from build123d import *

# Parameters (mm, degrees)
F0_R        = 72.39
F1_DEPTH    = 6.35
F2_DEPTH    = 50.8
F3_T1_DEPTH = 69.85
F5_DEPTH    = 31.75


# Not quite as in the source:
# - a fillet or chamfer that OpenCascade refuses, or shapes differently, is made with other operations: its cross-section is extruded or revolved along the edge and cut away or added


with BuildPart() as f1:
    # F0 (on Top) → F1 (new body)
    with BuildSketch(Plane.XY):
        with BuildLine():
            Line((38.1, -87.9881810245), (50.8, -87.9881810245))
            Line((50.8, -87.9881810245), (57.15, -76.9896583964))
            ThreePointArc((57.15, -76.9896583964), (109.1955678842, -63.0440905122), (95.25, -10.9985226281))
            Line((95.25, -10.9985226281), (101.6, 0))
            Line((101.6, 0), (95.25, 10.9985226281))
            ThreePointArc((95.25, 10.9985226281), (109.1955678842, 63.0440905122), (57.15, 76.9896583964))
            Line((57.15, 76.9896583964), (50.8, 87.9881810245))
            Line((50.8, 87.9881810245), (38.1, 87.9881810245))
            ThreePointArc((38.1, 87.9881810245), (0, 126.0881810245), (-38.1, 87.9881810245))
            Line((-38.1, 87.9881810245), (-50.8, 87.9881810245))
            Line((-50.8, 87.9881810245), (-57.15, 76.9896583964))
            ThreePointArc((-57.15, 76.9896583964), (-109.1955678842, 63.0440905122), (-95.25, 10.9985226281))
            Line((-95.25, 10.9985226281), (-101.6, 0))
            Line((-101.6, 0), (-95.25, -10.9985226281))
            ThreePointArc((-95.25, -10.9985226281), (-109.1955678842, -63.0440905122), (-57.15, -76.9896583964))
            Line((-57.15, -76.9896583964), (-50.8, -87.9881810245))
            Line((-50.8, -87.9881810245), (-38.1, -87.9881810245))
            ThreePointArc((-38.1, -87.9881810245), (0, -126.0881810245), (38.1, -87.9881810245))
        make_face()
        Circle(F0_R, mode=Mode.SUBTRACT)
    extrude(amount=F1_DEPTH)

    # F0 (on Top) → F2 (join)
    with BuildSketch(Plane.XY):
        Circle(F0_R)
    extrude(amount=F2_DEPTH)

    # F3: fillet of radius 38.1 on 6 edges, made by hand

    # F3_s2 → F3_t1 (cut)
    with BuildSketch(Plane.XY.offset(-31.75)):
        with BuildLine():
            ThreePointArc((57.15, 76.9896583964), (48.4360135972, 83.8936364665), (38.1, 87.9881810245))
            Line((38.1, 87.9881810245), (50.8, 87.9881810245))
            Line((50.8, 87.9881810245), (57.15, 76.9896583964))
        make_face()
        with BuildLine():
            ThreePointArc((95.25, -10.9985226281), (96.8720271945, 0), (95.25, 10.9985226281))
            Line((95.25, 10.9985226281), (101.6, 0))
            Line((101.6, 0), (95.25, -10.9985226281))
        make_face()
        with BuildLine():
            ThreePointArc((38.1, -87.9881810245), (48.4360135972, -83.8936364665), (57.15, -76.9896583964))
            Line((57.15, -76.9896583964), (50.8, -87.9881810245))
            Line((50.8, -87.9881810245), (38.1, -87.9881810245))
        make_face()
        with BuildLine():
            ThreePointArc((-38.1, -87.9881810245), (-48.4360135972, -83.8936364665), (-57.15, -76.9896583964))
            Line((-57.15, -76.9896583964), (-50.8, -87.9881810245))
            Line((-50.8, -87.9881810245), (-38.1, -87.9881810245))
        make_face()
        with BuildLine():
            ThreePointArc((-95.25, 10.9985226281), (-96.8720271945, 0), (-95.25, -10.9985226281))
            Line((-95.25, -10.9985226281), (-101.6, 0))
            Line((-101.6, 0), (-95.25, 10.9985226281))
        make_face()
        with BuildLine():
            ThreePointArc((-38.1, 87.9881810245), (-48.4360135972, 83.8936364665), (-57.15, 76.9896583964))
            Line((-57.15, 76.9896583964), (-50.8, 87.9881810245))
            Line((-50.8, 87.9881810245), (-38.1, 87.9881810245))
        make_face()
    extrude(amount=F3_T1_DEPTH, mode=Mode.SUBTRACT)

    # F4 (on face) → F5 (join)
    with BuildSketch(Plane.XY.offset(6.35)):
        with BuildLine():
            ThreePointArc((-95.25, -10.9985226281), (-109.1955678842, -63.0440905122), (-57.15, -76.9896583964))
            ThreePointArc((-57.15, -76.9896583964), (-48.4360135972, -83.8936364665), (-38.1, -87.9881810245))
            ThreePointArc((-38.1, -87.9881810245), (0, -126.0881810245), (38.1, -87.9881810245))
            ThreePointArc((38.1, -87.9881810245), (48.4360135972, -83.8936364665), (57.15, -76.9896583964))
            ThreePointArc((57.15, -76.9896583964), (109.1955678842, -63.0440905122), (95.25, -10.9985226281))
            ThreePointArc((95.25, -10.9985226281), (96.8720271945, 0), (95.25, 10.9985226281))
            ThreePointArc((95.25, 10.9985226281), (109.1955678842, 63.0440905122), (57.15, 76.9896583964))
            ThreePointArc((57.15, 76.9896583964), (48.4360135972, 83.8936364665), (38.1, 87.9881810245))
            ThreePointArc((38.1, 87.9881810245), (0, 126.0881810245), (-38.1, 87.9881810245))
            ThreePointArc((-38.1, 87.9881810245), (-48.4360135972, 83.8936364665), (-57.15, 76.9896583964))
            ThreePointArc((-57.15, 76.9896583964), (-109.1955678842, 63.0440905122), (-95.25, 10.9985226281))
            ThreePointArc((-95.25, 10.9985226281), (-96.8720271945, 0), (-95.25, -10.9985226281))
        make_face()
        with BuildLine():
            ThreePointArc((-92.7564557809, 13.2428401804), (-106.4459372272, 61.4565905122), (-57.8468639049, 73.7080269811))
            ThreePointArc((-57.8468639049, 73.7080269811), (-46.8485135972, 81.1440058095), (-34.909591876, 86.9508671615))
            ThreePointArc((-34.909591876, 86.9508671615), (0, 122.9131810245), (34.909591876, 86.9508671615))
            ThreePointArc((34.909591876, 86.9508671615), (46.8485135972, 81.1440058095), (57.8468639049, 73.7080269811))
            ThreePointArc((57.8468639049, 73.7080269811), (106.4459372272, 61.4565905122), (92.7564557809, 13.2428401804))
            ThreePointArc((92.7564557809, 13.2428401804), (93.6970271945, 0), (92.7564557809, -13.2428401804))
            ThreePointArc((92.7564557809, -13.2428401804), (106.4459372272, -61.4565905122), (57.8468639049, -73.7080269811))
            ThreePointArc((57.8468639049, -73.7080269811), (46.8485135972, -81.1440058095), (34.909591876, -86.9508671615))
            ThreePointArc((34.909591876, -86.9508671615), (0, -122.9131810245), (-34.909591876, -86.9508671615))
            ThreePointArc((-34.909591876, -86.9508671615), (-46.8485135972, -81.1440058095), (-57.8468639049, -73.7080269811))
            ThreePointArc((-57.8468639049, -73.7080269811), (-106.4459372272, -61.4565905122), (-92.7564557809, -13.2428401804))
            ThreePointArc((-92.7564557809, -13.2428401804), (-93.6970271945, 0), (-92.7564557809, 13.2428401804))
        make_face(mode=Mode.SUBTRACT)
    extrude(amount=F5_DEPTH)


solid = f1.part
Geometry: final body of the model. Coordinates: model frame, mm. A direction names the side the tool comes from. Coordinates: 2 decimals unless noted, no trailing zeros. Order: outer loops, then holes, each group sorted by start corner. A loop starts at its lowest first (then second) coordinate and runs counter-clockwise, first axis right, second up.
(1) Section query B-B (y = 0). Return the cut outline in (x, z).
(2) Material intervals for probe 1 along Y at (x, z) = (47.5, 31); probe 2 along Y at (x, z) = (21, 25); probe 3 along Z at (x, y) = (10, -113.5), sorted ascending.
(3) Section query A-A (z = 16.5). Return the cut outline in (x, y) (3 decimals), plus the area to 3 significant figures.
(4) First-contact query: pin 1 (1.5 mm diameter, centred on x = 65, z = 36, fed in from -Y); pin 2 (4 mm diameter, centred on x = 29, z = 41, fed in from -Y); pin 3 (3 mm diameter, centred on x = 88, z = 12.5, fed in from +Y). Flat tips, straight axial feed; report the tip coordinate or a pass-through.
(5) Draft query along Y for faces 1 (the face through (0.84, 126.08, 18.78)), 2 (the face through (48.3, -83.97, 18.78)), 3 (the face through (-51, -53, 6.35)). Return one class per face: pulls with the +Y half, pulls with the -Y half, needs draft (parallel to the pull), parting line crosses it, or undercut.
(6) Access query for faces 4 (the face through (46.687, 81.237, 22.003)), 5 (the face through (48.6, 83.8, 18.8)), 6 (the face through (-96.87, 0.16, 18.78)). Directions: +Z, -Z, +X, -X, +Y, -Y. A direction counts if a zero-diameter tool reaches every point of the face in a straight line with its end or side. Return the directions, or none.
(7) Section query D-D (x = 0). Return the cut outline in (y, z), plus the area to 3 significant figures.
(8) Section query C-C (x = -76.2). Return the cut outline in (y, z), plus the area to 3 significant figures.
Solution:
1. outline: (-96.87, 0) - (96.87, 0) - (96.87, 38.1) - (93.7, 38.1) - (93.7, 6.35) - (72.39, 6.35) - (72.39, 50.8) - (-72.39, 50.8) - (-72.39, 6.35) - (-93.7, 6.35) - (-93.7, 38.1) - (-96.87, 38.1) - close
2. probe 1: y = -84.42 to -80.76, -54.63 to 54.63, 80.76 to 84.42
2. probe 2: y = -119.78 to -115.89, -69.28 to 69.28, 115.89 to 119.78
2. probe 3: z = 0 to 6.35
3. outline: (-95.25, -10.999) arc R38.1 ccw to (-57.15, -76.99) arc R38.1 ccw to (-38.1, -87.988) arc R38.1 ccw to (38.1, -87.988) arc R38.1 ccw to (57.15, -76.99) arc R38.1 ccw to (95.25, -10.999) arc R38.1 ccw to (95.25, 10.999) arc R38.1 ccw to (57.15, 76.99) arc R38.1 ccw to (38.1, 87.988) arc R38.1 ccw to (-38.1, 87.988) arc R38.1 ccw to (-57.15, 76.99) arc R38.1 ccw to (-95.25, 10.999) arc R38.1 ccw to start; circle Ø144.78 at (0, 0); hole (-92.756, -13.243) arc R34.925 ccw (long way) to (-57.847, -73.708) arc R93.697 ccw to (-34.91, -86.951) arc R34.925 ccw (long way) to (34.91, -86.951) arc R93.697 ccw to (57.847, -73.708) arc R34.925 ccw (long way) to (92.756, -13.243) arc R93.697 ccw to (92.756, 13.243) arc R34.925 ccw (long way) to (57.847, 73.708) arc R93.697 ccw to (34.91, 86.951) arc R34.925 ccw (long way) to (-34.91, 86.951) arc R93.697 ccw to (-57.847, 73.708) arc R34.925 ccw (long way) to (-92.756, 13.243) arc R93.697 ccw to start
3. area: 19,100 mm2
4. pin 1: stops at y = -80.63
4. pin 2: stops at y = -67.17
4. pin 3: stops at y = 80.68
5. face 1: pulls with the +Y half
5. face 2: pulls with the -Y half
5. face 3: undercut
6. face 4: +Z
6. face 5: +Z, -Z, +Y
6. face 6: +Z, -Z, -X
7. outline: (-126.09, 0) - (126.09, 0) - (126.09, 38.1) - (122.91, 38.1) - (122.91, 6.35) - (72.39, 6.35) - (72.39, 50.8) - (-72.39, 50.8) - (-72.39, 6.35) - (-122.91, 6.35) - (-122.91, 38.1) - (-126.09, 38.1) - close
7. area: 8,240 mm2
8. outline: (-82.09, 0) - (82.09, 0) - (82.09, 38.1) - (78.92, 38.1) - (78.92, 6.35) - (-78.92, 6.35) - (-78.92, 38.1) - (-82.09, 38.1) - close
8. area: 1,240 mm2
